```python
from build123d import *

# Parameters (mm, degrees)
SKETCH_1_R          = 10
SKETCH_1_R_2        = 1.25
EXTRUDE_1_DEPTH     = 2
SKETCH_2_R          = 4.5
EXTRUDE_2_DEPTH     = 2
SKETCH_3_R          = 2.5
CUT_EXTRUDE_1_DEPTH = 2


with BuildPart() as part:
    # 草图1 → 凸台-拉伸1 (new body)
    with BuildSketch(Plane(origin=(0, 0, 0), x_dir=(1, 0, 0), z_dir=(0, 1, 0))):
        with Locations(Location((0, 0, 0), (0, 0, 270))):
            Circle(SKETCH_1_R)
        with Locations(Location((0, 6.5, 0), (0, 0, 270))):
            Circle(SKETCH_1_R_2, mode=Mode.SUBTRACT)
        with Locations(Location((6.5, 0, 0), (0, 0, 270))):
            Circle(SKETCH_1_R_2, mode=Mode.SUBTRACT)
        with Locations(Location((0, -6.5, 0), (0, 0, 270))):
            Circle(SKETCH_1_R_2, mode=Mode.SUBTRACT)
        with Locations(Location((-6.5, 0, 0), (0, 0, 270))):
            Circle(SKETCH_1_R_2, mode=Mode.SUBTRACT)
    extrude(amount=EXTRUDE_1_DEPTH)

    # 草图2 → 凸台-拉伸2 (add)
    with BuildSketch(Plane.XZ):
        with Locations(Location((0, 0, 0), (0, 0, 270))):
            Circle(SKETCH_2_R)
    extrude(amount=EXTRUDE_2_DEPTH)

    # 草图3 → 切除-拉伸1 (cut)
    with BuildSketch(Plane.XZ.offset(2)):
        with Locations(Location((0, 0, 0), (0, 0, 270))):
            Circle(SKETCH_3_R)
    extrude(amount=-CUT_EXTRUDE_1_DEPTH, mode=Mode.SUBTRACT)


solid = part.part
```
Model file for the job. Use its own axes, mm. A direction names the side the tool comes from. Give positions to 0.01 mm unless a question says otherwise; leave off trailing zeros. Write each loop counter-clockwise with the first axis right and the second up, starting at its lowest first coordinate (ties: lowest second). Pieces come first, ordered by that corner, then holes. Notation, with made-up numbers: (18.25, 28) - (33.25, 28) arc R31 cw to (33.25, 66) - close; hole circle Ø5 at (24, -13.75). An arc over 180 degrees is marked (long way). One line per question, with ' | ' between items. Start each with the question number.
(1) Slice it at D-D on z = 7.25. Write the cut outline in (x, y), plus the area to 4 significant figures.
(2) Two-plate mould, pull along X, no slides. Class faces 3 (the face through (-9.76, 0.99, -2.17)), 4 (the face through (5.28, 0.99, -0.27)), 5 (the face through (0, 2, 0)): +X half, -X half, draft (parallel to the pull), parting line (faces both ways), or undercut.
(3) Pin check, flat tips, straight feed: P1, Ø1.5, axis at x = 0, z = -6.5, coming from the +Y side; P2, Ø2.5, axis at x = -1, z = 0, coming from the -Y side; P3, Ø2, axis at y = 1, z = -2.5, coming from the +X side. Stop position of each tip, or through.
(4) Slice it at C-C on x = 6.5. Write the cut outline in (y, z).
(5) Slice it at B-B on x = 0. Write the cut outline in (y, z), plus the area to 3 significant figures.
(6) Wall check: line 1 along X through (y, z) = (1.1, 0); line 2 along Z through (x, y) = (1, 1.05); line 3 along Y through (x, z) = (5, -7.25). Give the ranges that are in metal, low to high. Write a range as from..to.
(7) Slice it at A-A on z = 0. Write the cut outline in (x, y).
(8) 3-axis set-ups, long thin cutter, end or side, ignore diameter. For faces 1 (the face through (0, 0, 0)), 2 (the face through (-7.72, 0.99, -0.27)): which of +Z, -Z, +X, -X, +Y, -Y reach the whole face in a straight line?
Results below:
1) outline: (-6.89, 0) - (-1, 0) - (-1, 2) - (-6.89, 2) - close; (1, 0) - (6.89, 0) - (6.89, 2) - (1, 2) - close | area: 23.55 mm^2
2) face 3: parting line | face 4: undercut | face 5: draft
3) P1: through | P2: y = 0 | P3: x = 9.89
4) outline: (0, -7.6) - (2, -7.6) - (2, -1.25) - (0, -1.25) - close; (0, 1.25) - (2, 1.25) - (2, 7.6) - (0, 7.6) - close
5) outline: (-2, -4.5) - (0, -4.5) - (0, -5.25) - (2, -5.25) - (2, 5.25) - (0, 5.25) - (0, 4.5) - (-2, 4.5) - (-2, 2.5) - (0, 2.5) - (0, -2.5) - (-2, -2.5) - close; (0, -10) - (2, -10) - (2, -7.75) - (0, -7.75) - close; (0, 7.75) - (2, 7.75) - (2, 10) - (0, 10) - close | area: 38.0 mm^2
6) line 1: -10..-7.75, -5.25..5.25, 7.75..10 | line 2: -9.95..-7.25, -5.75..5.75, 7.25..9.95 | line 3: 0..2
7) outline: (-10, 0) - (-7.75, 0) - (-7.75, 2) - (-10, 2) - close; (-5.25, 0) - (-4.5, 0) - (-4.5, -2) - (-2.5, -2) - (-2.5, 0) - (2.5, 0) - (2.5, -2) - (4.5, -2) - (4.5, 0) - (5.25, 0) - (5.25, 2) - (-5.25, 2) - close; (7.75, 0) - (10, 0) - (10, 2) - (7.75, 2) - close
8) face 1: -Y | face 2: +Y, -Y
